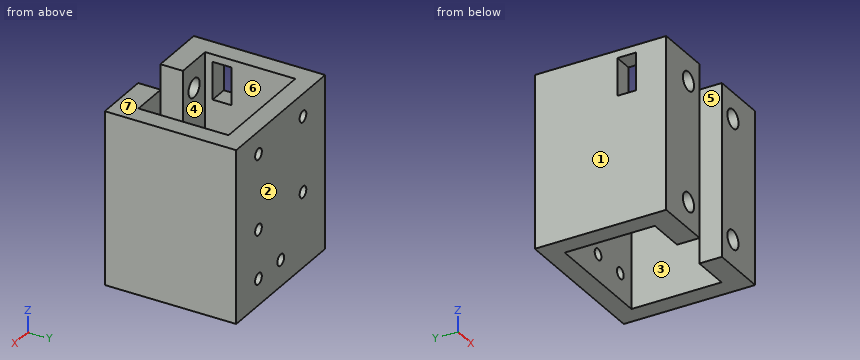
```python
from build123d import *

# Parameters (mm, degrees)
BOSS_EXTRUDE1_DEPTH = 46
SKETCH2_R           = 2.5
CUT_EXTRUDE1_DEPTH  = 6
SKETCH3_R           = 1.5
CUT_EXTRUDE2_DEPTH  = 5
SKETCH4_R           = 1.5
CUT_EXTRUDE3_DEPTH  = 5
SKETCH5_W           = 10
SKETCH5_H           = 5
CUT_EXTRUDE4_DEPTH  = 5


with BuildPart() as part:
    # Sketch1 → Boss-Extrude1 (new body)
    with BuildSketch(Plane.XY):
        Polygon((20, 39.058190014), (-20, 39.058190014), (-20, 4.058190014), (-5, 4.058190014), (-5, 10.058190014), (-15, 10.058190014), (-15, 34.058190014), (15, 34.058190014), (15, 10.058190014), (5, 10.058190014), (5, 4.058190014), (20, 4.058190014), align=None)
    extrude(amount=BOSS_EXTRUDE1_DEPTH)

    # Sketch2 → Cut-Extrude1 (cut)
    with BuildSketch(Plane(origin=(0, 4.058190014, 0), x_dir=(-1, 0, 0), z_dir=(0, -1, 0))):
        with Locations(Location((10, -39, 0), (0, 0, 180))):
            Circle(SKETCH2_R)
        with Locations(Location((-10, -39, 0), (0, 0, 180))):
            Circle(SKETCH2_R)
        with Locations(Location((-10, -7, 0), (0, 0, 180))):
            Circle(SKETCH2_R)
        with Locations(Location((10, -7, 0), (0, 0, 180))):
            Circle(SKETCH2_R)
    extrude(amount=-CUT_EXTRUDE1_DEPTH, mode=Mode.SUBTRACT)

    # Sketch3 → Cut-Extrude2 (cut)
    with BuildSketch(Plane(origin=(0, 39.058190014, 0), x_dir=(1, 0, 0), z_dir=(0, 1, 0))):
        with Locations(Location((-10, -20, 0), (0, 0, 180))):
            Circle(SKETCH3_R)
        with Locations(Location((10, -20, 0), (0, 0, 180))):
            Circle(SKETCH3_R)
        with Locations(Location((-10, -40, 0), (0, 0, 180))):
            Circle(SKETCH3_R)
        with Locations(Location((10, -40, 0), (0, 0, 180))):
            Circle(SKETCH3_R)
    extrude(amount=-CUT_EXTRUDE2_DEPTH, mode=Mode.SUBTRACT)

    # Sketch4 → Cut-Extrude3 (cut)
    with BuildSketch(Plane(origin=(0, 39.058190014, 0), x_dir=(1, 0, 0), z_dir=(0, 1, 0))):
        with Locations(Location((10, -7, 0), (0, 0, 180))):
            Circle(SKETCH4_R)
        with Locations(Location((0, -7, 0), (0, 0, 180))):
            Circle(SKETCH4_R)
    extrude(amount=-CUT_EXTRUDE3_DEPTH, mode=Mode.SUBTRACT)

    # Sketch5 → Cut-Extrude4 (cut)
    with BuildSketch(Plane.ZY.offset(20)):
        with Locations((39, 14.558190014)):
            Rectangle(SKETCH5_W, SKETCH5_H)
    extrude(amount=-CUT_EXTRUDE4_DEPTH, mode=Mode.SUBTRACT)


solid = part.part
```
CAD build for the part. Positions are in the model's coordinates, mm. Face numbers are marked on the shaded views. A direction names the side the tool comes from. Round coordinates to 2 decimals unless told otherwise and drop trailing zeros. Order: outer loops, then holes, each group sorted by start corner. A loop starts at its lowest first (then second) coordinate and runs counter-clockwise, first axis right, second up. Notation, with made-up numbers: (-20, 5.25) -> (24, 5.25) arc R29 cw to (24, 31.25) -> close; hole circle Ø11 at (43, 70). An arc over 180 degrees is marked (long way). One line per question, with ' | ' between items.
Q1. Slice it at B-B (x = 10). Write the cut outline in (y, z), then the cut area to 3 significant figures.
Completed:
outline: (4.06, 0) -> (10.06, 0) -> (10.06, 4.5) -> (4.06, 4.5) -> close; (4.06, 9.5) -> (10.06, 9.5) -> (10.06, 36.5) -> (4.06, 36.5) -> close; (4.06, 41.5) -> (10.06, 41.5) -> (10.06, 46) -> (4.06, 46) -> close; (34.06, 0) -> (39.06, 0) -> (39.06, 5.5) -> (34.06, 5.5) -> close; (34.06, 8.5) -> (39.06, 8.5) -> (39.06, 18.5) -> (34.06, 18.5) -> close; (34.06, 21.5) -> (39.06, 21.5) -> (39.06, 38.5) -> (34.06, 38.5) -> close; (34.06, 41.5) -> (39.06, 41.5) -> (39.06, 46) -> (34.06, 46) -> close | area: 401 mm^2
Q2. Slice it at A-A (y = 15). Write the cut outline in (x, z), then the cut area to 3 significant figures.
Completed:
outline: (-20, 0) -> (-15, 0) -> (-15, 34) -> (-20, 34) -> close; (-20, 44) -> (-15, 44) -> (-15, 46) -> (-20, 46) -> close; (15, 0) -> (20, 0) -> (20, 46) -> (15, 46) -> close | area: 410 mm^2
Q3. Which spindle directions (+Z, -Z, +X, -X, +Y, -Y) get a long thin tool onto all of the face, cutting with end or side? Do the marked faces 5, 6 and 7. Say none if no direction does.
Completed:
face 5: +Z, -Z, -Y | face 6: +Z, -Z | face 7: +Z, +X, -X, +Y, -Y
Q4. Two-plate mould, pull along Y, no slides. Class the marked faces 1, 2, 3 and 4: released by +Y, released by -Y, zero draft, split by the parting line, or undercut.
Completed:
face 1: zero draft | face 2: released by +Y | face 3: undercut | face 4: undercut
Q5. Slice it at C-C (z = 7). Write the cut outline in (x, y), then the cut area to 3 significant figures.
Completed:
outline: (-20, 4.06) -> (-12.5, 4.06) -> (-12.5, 10.06) -> (-15, 10.06) -> (-15, 34.06) -> (-1.5, 34.06) -> (-1.5, 39.06) -> (-20, 39.06) -> close; (-7.5, 4.06) -> (-5, 4.06) -> (-5, 10.06) -> (-7.5, 10.06) -> close; (1.5, 34.06) -> (8.5, 34.06) -> (8.5, 39.06) -> (1.5, 39.06) -> close; (5, 4.06) -> (7.5, 4.06) -> (7.5, 10.06) -> (5, 10.06) -> close; (11.5, 34.06) -> (15, 34.06) -> (15, 10.06) -> (12.5, 10.06) -> (12.5, 4.06) -> (20, 4.06) -> (20, 39.06) -> (11.5, 39.06) -> close | area: 530 mm^2
Q6. Drop a flat-ended pin along its axis: pin 1 (1.8 mm diameter, centred on x = 0, z = 7, fed in from +Y). Give the stop position or say it passes through.
Completed:
pin 1: passes through
Q7. Slice it at D-D (x = 0). Write the cut outline in (y, z).
Completed:
outline: (34.06, 0) -> (39.06, 0) -> (39.06, 5.5) -> (34.06, 5.5) -> close; (34.06, 8.5) -> (39.06, 8.5) -> (39.06, 46) -> (34.06, 46) -> close
Q8. Probe probe 1 along Z at (x, y) = (10, 8.75); probe 2 along X at (y, z) = (26.5, 30.5); probe 3 along Z at (x, y) = (0, 36.1). List the from-to ranges inside material, lowest first.
Completed:
probe 1: z = 0 to 4.5, 9.5 to 36.5, 41.5 to 46 | probe 2: x = -20 to -15, 15 to 20 | probe 3: z = 0 to 5.5, 8.5 to 46
